Here's how the part is built. I have some questions about the finished solid (model axes, mm). Give positions to 0.01 mm unless a question says otherwise; leave off trailing zeros. Loops run counter-clockwise (first coordinate to the right, second up) from the corner with the lowest first, then second, coordinate; pieces in that order, holes last.
Q1. If we section it at B-B (x = 18): Please give me the cut outline in (y, z).
Q2. If we section it at A-A (y = 0.4): Give the number of separate pieces and of enclosed holes in the cut face, plus the area to 3 significant figures.
Q3. I need wall thicknesses on line 1 (Z direction, x = 18.5, y = 1.85); line 2 (X direction, y = 1.7, z = -7.5); line 3 (Z direction, x = -3, y = 0.9). Which ranges of each line are inside material? Lowest first, please.
Q4. Will these pins go through, and if not, where does the flat tip stop? P1, Ø5, axis at x = 1, z = 6, coming from the -Y side; P2, Ø2.5, axis at x = 7.63, z = 18.49, coming from the +Y side; P3, Ø7, axis at x = 3.64, z = -6.56, coming from the -Y side.
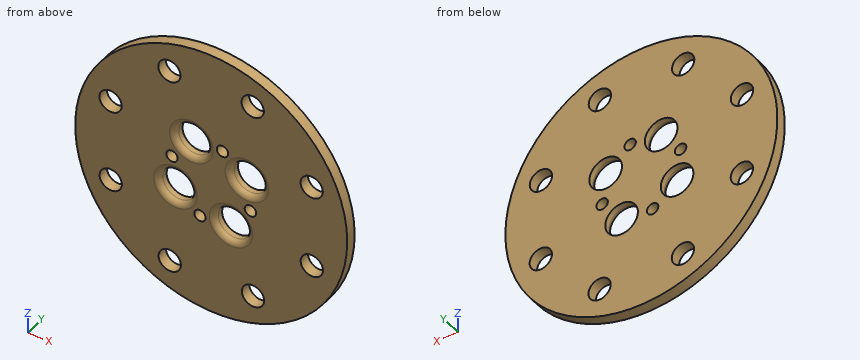
from build123d import *

# Parameters (mm, degrees)
SKETCH1_R           = 25
BOSS_EXTRUDE1_DEPTH = 2
SKETCH2_R           = 1.05
SKETCH2_R_2         = 3
CUT_EXTRUDE1_DEPTH  = 3
FILLET1_R           = 1
SKETCH4_R           = 2.05
CUT_EXTRUDE3_DEPTH  = 3


with BuildPart() as part:
    # Sketch1 → Boss-Extrude1 (new body)
    with BuildSketch(Plane(origin=(0, 0, 0), x_dir=(1, 0, 0), z_dir=(0, 1, 0))):
        Circle(SKETCH1_R)
    extrude(amount=BOSS_EXTRUDE1_DEPTH)

    # Sketch2 → Cut-Extrude1 (cut, through all)
    with BuildSketch(Plane(origin=(0, 2, 0), x_dir=(1, 0, 0), z_dir=(0, 1, 0))):
        with Locations((-2.066368974, 7.209723938)):
            Circle(SKETCH2_R)
        with Locations((7.209723938, 2.066368974)):
            Circle(SKETCH2_R)
        with Locations((2.066368974, -7.209723938)):
            Circle(SKETCH2_R)
        with Locations((-7.209723938, -2.066368974)):
            Circle(SKETCH2_R)
        with Locations((-3.636901173, -6.559188201)):
            Circle(SKETCH2_R_2)
        with Locations((-6.559188201, 3.636901173)):
            Circle(SKETCH2_R_2)
        with Locations((3.636901173, 6.559188201)):
            Circle(SKETCH2_R_2)
        with Locations((6.559188201, -3.636901173)):
            Circle(SKETCH2_R_2)
    extrude(amount=-CUT_EXTRUDE1_DEPTH, mode=Mode.SUBTRACT)

    # Fillet1
    fillet1_edges = [part.edges().sort_by_distance(p)[0] for p in [
        (-6.636901173, 0, 6.559188201),
        (-9.559188201, 0, -3.636901173),
        (0.636901173, 0, -6.559188201),
        (3.559188201, 0, 3.636901173),
    ]]
    fillet(fillet1_edges, radius=FILLET1_R)

    # Sketch4 → Cut-Extrude3 (cut, through all)
    with BuildSketch(Plane.XZ):
        with Locations((-18.488747294, 7.626678405)):
            Circle(SKETCH4_R)
        with Locations((-7.680642569, 18.466394605)):
            Circle(SKETCH4_R)
        with Locations((7.626678405, 18.488747294)):
            Circle(SKETCH4_R)
        with Locations((18.466394605, 7.680642569)):
            Circle(SKETCH4_R)
        with Locations((18.488747294, -7.626678405)):
            Circle(SKETCH4_R)
        with Locations((7.680642569, -18.466394605)):
            Circle(SKETCH4_R)
        with Locations((-7.626678405, -18.488747294)):
            Circle(SKETCH4_R)
        with Locations((-18.466394605, -7.680642569)):
            Circle(SKETCH4_R)
    extrude(amount=-CUT_EXTRUDE3_DEPTH, mode=Mode.SUBTRACT)


solid = part.part
Check sheet entries:
1. outline: (0, -17.35) - (2, -17.35) - (2, -9.62) - (0, -9.62) - close; (0, -5.64) - (2, -5.64) - (2, 5.68) - (0, 5.68) - close; (0, 9.68) - (2, 9.68) - (2, 17.35) - (0, 17.35) - close
2. separate pieces: 1
2. enclosed holes: 16
2. area: 1,720 mm2
3. line 1: z = -16.82 to -9.68, -5.58 to 5.63, 9.73 to 16.82
3. line 2: x = -23.85 to -20.51, -16.42 to -3.08, -1.06 to 0.79, 6.49 to 16.44, 20.53 to 23.85
3. line 3: z = -24.82 to -7.69, -6.73 to 3.62, 9.5 to 24.82
4. P1: stops at y = 0
4. P2: passes through
4. P3: stops at y = 0.13
